Geometry: final body of the model. Coordinates: model frame, mm. Face numbers are marked on the shaded views. A direction names the side the tool comes from. Round coordinates to 2 decimals unless told otherwise and drop trailing zeros. Order: outer loops, then holes, each group sorted by start corner. A loop starts at its lowest first (then second) coordinate and runs counter-clockwise, first axis right, second up. Notation, with made-up numbers: (33.25, 81) -> (88.25, 81) arc R25 cw to (88.25, 108) -> close; hole circle Ø5 at (71.25, -27.5). An arc over 180 degrees is marked (long way). Put each result on its own line as item: value.
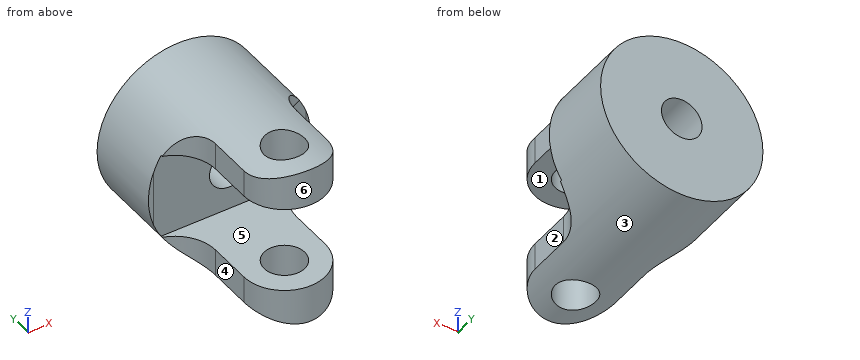
```python
from build123d import *

# Parameters (mm, degrees)
SKETCH1_R               = 19.05
BASE_EXTRUDE_DEPTH      = 47.625
CUT_EXTRUDE1_DEPTH      = 20.05
CUT_EXTRUDE1_DEPTH_BACK = 20.05
CUT_EXTRUDE5_DEPTH      = 20.0500001
CUT_EXTRUDE5_DEPTH_BACK = 20.0500001
SKETCH11_R              = 4.7625
CUT_EXTRUDE6_DEPTH      = 20.0500001
CUT_EXTRUDE6_DEPTH_BACK = 20.0500001
SKETCH12_R              = 4.7625
CUT_EXTRUDE7_DEPTH      = 48.625000104


with BuildPart() as part:
    # Sketch1 → Base-Extrude (new body)
    with BuildSketch(Plane(origin=(0, 0, 0), x_dir=(-1, 0, 0), z_dir=(0, 1, 0))):
        Circle(SKETCH1_R)
    extrude(amount=BASE_EXTRUDE_DEPTH)

    # Sketch2 → Cut-Extrude1 (cut, two sides)
    with BuildSketch(Plane.XY) as cut_extrude1_sk:
        with BuildLine():
            Line((-19.05, -131.979516723), (-19.05, 0))
            Line((-19.05, 0), (-19.05, 29.21))
            ThreePointArc((-19.05, 29.21), (-12.314807909, 26.420192091), (-9.525, 19.685))
            Line((-9.525, 19.685), (-9.525, 9.525))
            ThreePointArc((-9.525, 9.525), (0, 0), (9.525, 9.525))
            Line((9.525, 9.525), (9.525, 19.685))
            ThreePointArc((9.525, 19.685), (12.314807909, 26.420192091), (19.05, 29.21))
            Line((19.05, 29.21), (19.05, 0))
            Line((19.05, 0), (19.05, -131.979516723))
            Line((19.05, -131.979516723), (19.05, -395.938550169))
            Line((19.05, -395.938550169), (-19.05, -395.938550169))
            Line((-19.05, -395.938550169), (-19.05, -131.979516723))
        make_face()
    extrude(amount=CUT_EXTRUDE1_DEPTH, mode=Mode.SUBTRACT)
    extrude(cut_extrude1_sk.sketch, amount=-CUT_EXTRUDE1_DEPTH_BACK, mode=Mode.SUBTRACT)

    # Sketch8 → Cut-Extrude5 (cut, two sides)
    with BuildSketch(Plane(origin=(0, 0, 0), x_dir=(0, 0, -1), z_dir=(1, 0, 0))) as cut_extrude5_sk:
        Polygon((-10.16, -121.738350451), (-10.16, 0), (-10.16, 29.145238826), (10.16, 29.145238826), (10.16, 0), (10.16, -121.738350451), (10.16, -365.215051352), (-10.16, -365.215051352), align=None)
    extrude(amount=CUT_EXTRUDE5_DEPTH, mode=Mode.SUBTRACT)
    extrude(cut_extrude5_sk.sketch, amount=-CUT_EXTRUDE5_DEPTH_BACK, mode=Mode.SUBTRACT)

    # Sketch11 → Cut-Extrude6 (cut, two sides)
    with BuildSketch(Plane.XY) as cut_extrude6_sk:
        with Locations((0, 9.525)):
            Circle(SKETCH11_R)
    extrude(amount=CUT_EXTRUDE6_DEPTH, mode=Mode.SUBTRACT)
    extrude(cut_extrude6_sk.sketch, amount=-CUT_EXTRUDE6_DEPTH_BACK, mode=Mode.SUBTRACT)

    # Sketch12 → Cut-Extrude7 (cut, through all)
    with BuildSketch(Plane(origin=(0, 47.625, 0), x_dir=(-1, 0, 0), z_dir=(0, 1, 0))):
        Circle(SKETCH12_R)
    extrude(amount=-CUT_EXTRUDE7_DEPTH, mode=Mode.SUBTRACT)


solid = part.part
```
1. Cut plane D-D on x = -7. Return loops of the section in (y, z) (3 decimals), and give its area (3 significant figures).
Ans:
outline: (3.065, -17.717) -> (47.625, -17.717) -> (47.625, 17.717) -> (3.065, 17.717) -> (3.065, 10.16) -> (29.145, 10.16) -> (29.145, -10.16) -> (3.065, -10.16) -> close
area: 1,050 mm²
2. Contact query for flat-ended pins moving along their axis: P1, Ø8, axis at y = 12, z = -9, coming from the -X side (3 decimals); P2, Ø10, axis at x = 6.5, z = -3.5, coming from the -Y side; P3, Ø7, axis at y = 12, z = -12.5, coming from the +X side (3 decimals). Output: stop coordinate, or through.
Ans:
P1: x = -9.525
P2: y = 29.15
P3: x = 9.525
3. Material intervals for probe 1 along Y at (x, z) = (0, -15.75) (1 decimal); probe 2 along Z at (x, y) = (0, 34.25); probe 3 along Z at (x, y) = (11, 28), sorted ascending.
Ans:
probe 1: 0 to 4.8, 14.3 to 47.6
probe 2: -19.05 to -4.76, 4.76 to 19.05
probe 3: -15.55 to -10.16, 10.16 to 15.55
4. Cut plane A-A on x = 0. State how many separate pieces and enclosed holes the cut face has, and give its area (3 significant figures).
Ans:
separate pieces: 4
enclosed holes: 0
area: 877 mm²
5. Set-up query: the marked faces 4, 5 and 6. Return all of +Z, -Z, +X, -X, +Y, -Y with unobstructed straight access to the full face (end or side cutting, diameter ignored); none if empty.
Ans:
face 4: +Z, -Z, -X, -Y
face 5: +X, -X, -Y
face 6: +Z, -Z, -Y
6. Cut plane B-B on y = 6.5. Return loops of the section in (x, z).
Ans:
outline: (-9.03, -16.77) arc R19.05 ccw to (-3.68, -18.69) -> (-3.68, -10.16) -> (-9.03, -10.16) -> close; (-9.03, 10.16) -> (-3.68, 10.16) -> (-3.68, 18.69) arc R19.05 ccw to (-9.03, 16.77) -> close; (3.68, -18.69) arc R19.05 ccw to (9.03, -16.77) -> (9.03, -10.16) -> (3.68, -10.16) -> close; (3.68, 10.16) -> (9.03, 10.16) -> (9.03, 16.77) arc R19.05 ccw to (3.68, 18.69) -> close
7. Draft query along Z for the marked faces 1, 2 and 3. Return one class per face: +Z half, -Z half, draft (parallel to the pull), parting line (faces both ways), or undercut.
Ans:
face 1: undercut
face 2: draft
face 3: parting line
